Source: CAD feature listing. Evaluate the final solid. Frame: model axes, mm. A direction names the side the tool comes from. Round coordinates to 2 decimals unless told otherwise and drop trailing zeros. Loops run counter-clockwise (first coordinate to the right, second up) from the corner with the lowest first, then second, coordinate; pieces in that order, holes last. Notation, with made-up numbers: (16, 48.25) - (34, 48.25) arc R14 cw to (34, 52.25) - close; hole circle Ø10 at (-30.75, 87.5). An arc over 180 degrees is marked (long way). One line per question, with ' | ' between items. Start each with the question number.
1. Cut plane C-C (z = 4.5). Return loops of the section in (x, y), then the cut area to 3 significant figures.
2. Access query for faces 1 (the cylindrical face through (-1.5, -0.07, 34.96)), 2 (the flat face through (0, 0, 6)), 3 (the flat face through (1.3, -1.3, 0)). Directions: +Z, -Z, +X, -X, +Y, -Y. A direction counts if a zero-diameter tool reaches every point of the face in a straight line with its end or side. Return the directions, or none.
3. Ray query, line 1 (Y direction, x = 0, z = 4.6); line 2 (X direction, y = 1, z = 33); line 3 (Z direction, x = 0.25, y = 0.3). Return the intervals inside material, ascending.
4. Cut plane D-D (z = 17.5). Return loops of the section in (x, y), then the cut area to 3 significant figures.
5. Mould query, pull axis Y, two halves, no side actions, for faces 4 (the flat face through (0, 0, 32)), 5 (the cylindrical face through (-1.5, -0.07, 2.96)), 6 (the flat face through (1.3, -1.3, 38)), 7 (the cylindrical face through (-3, 0, 19)). Classes: pulls with the +Y half, pulls with the -Y half, needs draft (parallel to the pull), parting line crosses it, or undercut.
6. Pin query (flat end, axial travel): pin 1 (1.8 mm diameter, centred on x = 0, y = 0, fed in from -Z). Return the tip coordinate at first contact, or that it passes through.
7. Cut plane B-B (x = 0.95). Return loops of the section in (y, z), then the cut area to 3 significant figures.
8. Cut plane A-A (y = 0). Return loops of the section in (x, z).
Autodesk Inventor part; units mm, degrees
ref_plane "作業平面1" through (0, 0, 32) normal (0, 0, 1) x (1, 0, 0)
ref_plane "YZ Plane" through (0, 0, 0) normal (1, 0, 0) x (0, 1, 0)
ref_plane "XZ Plane" through (0, 0, 0) normal (0, 1, 0) x (-1, 0, 0)
sketch "スケッチ1" plane through (0, 0, 0) normal (0, 0, 1) x (1, 0, 0)
  circle A0 centre (0, 0) radius 1.5
  circle A1 centre (0, 0) radius 3
  dimension "d0" = 3
  dimension "d1" = 6
extrude "押し出し1" add sketch "スケッチ1" along normal blind 38
ref_plane "作業平面1" through (0, 0, 32) normal (0, 0, 1) x (1, 0, 0)
sketch "スケッチ3" plane through (0, 0, 32) normal (0, 0, 1) x (1, 0, 0)
  circle A0 centre (0, 0) radius 1.5
extrude "押し出し3" add sketch "スケッチ3" against normal blind 26
properties part number "スペーサーm3,38 自作" material "アルミニウム 7075"
Answers follow:
1) outline: circle Ø6 at (0, 0); hole circle Ø3 at (0, 0) | area: 21.2 mm2
2) face 1: +Z | face 2: -Z | face 3: -Z, +X, -X, +Y, -Y
3) line 1: y = -3 to -1.5, 1.5 to 3 | line 2: x = -2.83 to -1.12, 1.12 to 2.83 | line 3: z = 6 to 32
4) outline: circle Ø6 at (0, 0) | area: 28.3 mm2
5) face 4: undercut | face 5: undercut | face 6: needs draft | face 7: parting line crosses it
6) pin 1: stops at z = 6
7) outline: (-2.85, 0) - (-1.16, 0) - (-1.16, 6) - (1.16, 6) - (1.16, 0) - (2.85, 0) - (2.85, 38) - (1.16, 38) - (1.16, 32) - (-1.16, 32) - (-1.16, 38) - (-2.85, 38) - close | area: 188 mm2
8) outline: (-3, 0) - (-1.5, 0) - (-1.5, 6) - (1.5, 6) - (1.5, 0) - (3, 0) - (3, 38) - (1.5, 38) - (1.5, 32) - (-1.5, 32) - (-1.5, 38) - (-3, 38) - close
